Can you work these out from the model? Positions are in its coordinate system, mm. Round coordinates to 2 decimals unless told otherwise and drop trailing zeros. Order: outer loops, then holes, each group sorted by start corner. A loop starts at its lowest first (then second) coordinate and runs counter-clockwise, first axis right, second up. Notation, with made-up numbers: M 1.5,80.5 L 21.5,80.5 A28 ccw 21.5,102.5 Z; hole C 40,-38.75 d4. An arc over 180 degrees is marked long. One line per question, with ' | ' between items.
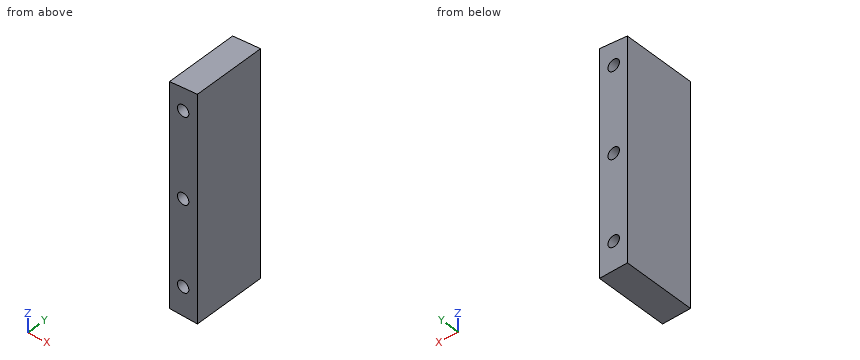
Autodesk Inventor part; units mm, degrees
ref_plane "YZ Plane" through (0, 0, 0) normal (1, 0, 0) x (0, 1, 0)
ref_plane "XZ Plane" through (0, 0, 0) normal (0, 1, 0) x (-1, 0, 0)
ref_plane "XY Plane" through (0, 0, 0) normal (0, 0, 1) x (1, 0, 0)
sketch "Sketch1" plane through (0, 0, 0) normal (0, 0, 1) x (1, 0, 0)
  line L0 (4.9, 12.6) -> (-4.9, 12.6)
  line L1 (-4.9, 12.6) -> (-4.9, -12.6)
  line L2 (-4.9, -12.6) -> (4.9, -12.6)
  line L3 (4.9, -12.6) -> (4.9, 12.6)
  line L4 (4.9, 12.6) -> (-4.9, -12.6) construction
  line L5 (-4.9, 12.6) -> (4.9, -12.6) construction
  point P0 (0, 0)
  dimension "d0" = 25.2
  dimension "d1" = 9.8
extrude "Extrusion1" add sketch "Sketch1" along normal blind 80
sketch "Sketch2" plane through (-4.9, 12.6, 0) normal (0, 1, 0) x (1, 0, 0)
  circle A0 centre (4.8, -70) radius 2
  circle A1 centre (4.8, -40) radius 2
  circle A2 centre (4.8, -10) radius 2
  line L0 (9.8, -80) -> (0, -80)
  line L1 (9.8, 0) -> (0, 0)
  line L2 (9.8, 0) -> (9.8, -80)
  point P0 (4.9, 0)
  point P1 (9.8, -40)
  dimension "d4" = 4
  dimension "d5" = 4
  dimension "d6" = 4
  dimension "d7" = 10
  dimension "d8" = 10
  dimension "d9" = 40
  dimension "d10" = 5
  dimension "d11" = 5
  dimension "d12" = 5
extrude "Extrusion2" cut sketch "Sketch2" against normal blind 80
sketch "Sketch3" plane through (-4.9, -12.6, 0) normal (0, -1, 0) x (1, 0, 0)
  arc A0 (48.1, 80) -> (-9.1978, 76.2369) centre (48.1, -358.1) ccw
  line L0 (0, 80) -> (9.8, 80)
  line L1 (0, 0) -> (0, 80)
  line L2 (0, 80) -> (48.1, 80)
  line L3 (-9.1978, 76.2369) -> (-9.1978, 80)
  line L4 (-9.1978, 80) -> (0, 80)
  point P0 (4.9, 0)
  point P1 (4.9, 80)
  dimension "d15" = 876.2
  dimension "d17" = 48.1
  dimension "d18" = 438.1
extrude "Extrusion3" cut sketch "Sketch3" against normal through all
properties part number "ReleaseMec2.0SideWall"
(1) If we section it at B-B on z = 10: Please give me the cut outline in (x, y).
Final values:
outline: M -4.9,-12.6 L -2.1,-12.6 L -2.1,12.6 L -4.9,12.6 Z; M 1.9,-12.6 L 4.9,-12.6 L 4.9,12.6 L 1.9,12.6 Z
(2) Will these pins go through, and if not, where does the flat tip stop? pin 1 Ø5 at (x, y) = (2, -4) entering from +Z; pin 2 Ø5 at (x, y) = (-2.5, 5) entering from +Z; pin 3 Ø2.5 at (x, z) = (-0.1, 70) entering from -Y.
Final values:
pin 1: z = 78.29 | pin 2: z = 77.86 | pin 3: through
(3) If we section it at C-C on x = -0.1: Please give me the cut outline in (y, z), plus the area to 3 significant figures.
Final values:
outline: M -12.6,0 L 12.6,0 L 12.6,8 L -12.6,8 Z; M -12.6,12 L 12.6,12 L 12.6,38 L -12.6,38 Z; M -12.6,42 L 12.6,42 L 12.6,68 L -12.6,68 Z; M -12.6,72 L 12.6,72 L 12.6,77.85 L -12.6,77.85 Z | area: 1,660 mm^2
(4) Please list where these lines run through material, in increasing order: probe 1 along X at (y, z) = (0.25, 70); probe 2 along Z at (x, y) = (-0.1, -5.5); probe 3 along Z at (x, y) = (-1, 9). Write a range as [from, to].
Final values:
probe 1: [-4.9, -2.1], [1.9, 4.9] | probe 2: [0, 8], [12, 38], [42, 68], [72, 77.85] | probe 3: [0, 8.21], [11.79, 38.21], [41.79, 68.21], [71.79, 77.76]
(5) If we section it at A-A on y = 10.5: Please give me the cut outline in (x, z).
Final values:
outline: M -4.9,0 L 4.9,0 L 4.9,78.32 A438.09 ccw -4.9,77.35 Z; hole C -0.1,10 d4; hole C -0.1,40 d4; hole C -0.1,70 d4
